The model under review builds one solid part; all positions refer to its coordinate system, in mm. A direction names the side the tool comes from. Coordinates: 2 decimals unless noted, no trailing zeros. Order: outer loops, then holes, each group sorted by start corner. A loop starts at its lowest first (then second) coordinate and runs counter-clockwise, first axis right, second up. Notation, with made-up numbers: M -19.75,-1.75 L 15.25,-1.75 A23 ccw 15.25,11.25 Z; hole C 87.25,44.25 d5. An arc over 180 degrees is marked long. Write each question's results on one line, items separated by ' | '.
from build123d import *

# Parameters (mm, degrees)
SKETCH1_W           = 170
SKETCH1_H           = 110
BOSS_EXTRUDE1_DEPTH = 30
FILLET2_R           = 10
FILLET3_R           = 10
FILLET4_R           = 10
SKETCH3_R           = 2.5
CUT_EXTRUDE1_DEPTH  = 5
CUT_EXTRUDE2_START  = -5
SKETCH5_R           = 2.5
CUT_EXTRUDE2_DEPTH  = 5
SKETCH6_W           = 3
SKETCH6_H           = 25
BOSS_EXTRUDE2_DEPTH = 25
SKETCH7_R           = 3.5
BOSS_EXTRUDE3_DEPTH = 4
SKETCH8_R           = 3.5
BOSS_EXTRUDE4_DEPTH = 4


with BuildPart() as part:
    # Sketch1 → Boss-Extrude1 (new body)
    with BuildSketch(Plane(origin=(0, 0, 0), x_dir=(1, 0, 0), z_dir=(0, 1, 0))):
        Rectangle(SKETCH1_W, SKETCH1_H)
    extrude(amount=BOSS_EXTRUDE1_DEPTH)

    # Fillet2
    fillet2_edges = [part.edges().sort_by_distance(p)[0] for p in [
        (-85, 30, 0),
        (0, 30, 55),
        (0, 0, 55),
        (85, 15, 55),
        (-85, 15, 55),
    ]]
    fillet(fillet2_edges, radius=FILLET2_R)

    # Fillet3
    # the kernel refuses this fillet: 10 mm, written as the material it takes off along each edge
    with BuildSketch(Plane(origin=(75, 20, 45), x_dir=(1, 0, 0), z_dir=(0, 1, 0))) as fillet3_piece_1_section:
        Polygon((0, 0), (FILLET3_R, 0), (FILLET3_R, -FILLET3_R), (0, -FILLET3_R), align=None)
    fillet3_piece_1 = extrude(amount=FILLET3_R, mode=Mode.PRIVATE)
    fillet3_piece_1 = fillet3_piece_1 - Plane(origin=(75, 20, 45), x_dir=(-0.7071067811865475, 0, -0.7071067811865475), z_dir=(0, 1, 0)) * Sphere(FILLET3_R, mode=Mode.PRIVATE)
    add(fillet3_piece_1, mode=Mode.SUBTRACT)
    with BuildSketch(Plane(origin=(75, 20, -45), x_dir=(0, 1, 0), z_dir=(0, 0, -1))) as fillet3_piece_2_section:
        Polygon((0, 0), (FILLET3_R, 0), (FILLET3_R, FILLET3_R), (0, FILLET3_R), align=None)
    fillet3_piece_2 = extrude(amount=FILLET3_R, mode=Mode.PRIVATE)
    fillet3_piece_2 = fillet3_piece_2 - Plane(origin=(75, 20, -45), x_dir=(-0.7071067811865475, -0.7071067811865475, 0), z_dir=(0, 0, -1)) * Sphere(FILLET3_R, mode=Mode.PRIVATE)
    add(fillet3_piece_2, mode=Mode.SUBTRACT)
    with BuildSketch(Plane(origin=(-85, -25, -55), x_dir=(1, 0, 0), z_dir=(0, 1, 0))) as fillet3_piece_3:
        with BuildLine():
            CenterArc((FILLET3_R, -FILLET3_R), FILLET3_R, 90, 90)
            Line((0, -FILLET3_R), (0, 0))
            Line((0, 0), (FILLET3_R, 0))
        make_face()
    extrude(amount=45, mode=Mode.SUBTRACT)
    with BuildSketch(Plane(origin=(85, 30, -45), x_dir=(-1, 0, 0), z_dir=(0, 0, 1))) as fillet3_piece_4:
        with BuildLine():
            CenterArc((FILLET3_R, FILLET3_R), FILLET3_R, 180, 90)
            Line((0, FILLET3_R), (0, 0))
            Line((0, 0), (FILLET3_R, 0))
        make_face()
    extrude(amount=90, mode=Mode.SUBTRACT)
    with BuildSketch(Plane(origin=(-75, 20, -55), x_dir=(-1, 0, 0), z_dir=(0, -1, 0))) as fillet3_piece_5:
        with BuildLine():
            CenterArc((10 - FILLET3_R, -FILLET3_R), FILLET3_R, 0, 90)
            Line((10, -FILLET3_R), (10, 0))
            Line((10, 0), (10 - FILLET3_R, 0))
        make_face()
    revolve(axis=Axis((-75, 20, -55), (0, 0, -1)), revolution_arc=90, mode=Mode.SUBTRACT)
    with BuildSketch(Plane(origin=(85, -25, -55), x_dir=(-1, 0, 0), z_dir=(0, 1, 0))) as fillet3_piece_6:
        with BuildLine():
            CenterArc((FILLET3_R, FILLET3_R), FILLET3_R, 180, 90)
            Line((0, FILLET3_R), (0, 0))
            Line((0, 0), (FILLET3_R, 0))
        make_face()
    extrude(amount=45, mode=Mode.SUBTRACT)
    with BuildSketch(Plane(origin=(-75, 30, -55), x_dir=(0, -1, 0), z_dir=(1, 0, 0))) as fillet3_piece_7:
        with BuildLine():
            CenterArc((FILLET3_R, -FILLET3_R), FILLET3_R, 90, 90)
            Line((0, -FILLET3_R), (0, 0))
            Line((0, 0), (FILLET3_R, 0))
        make_face()
    extrude(amount=150, mode=Mode.SUBTRACT)

    # Fillet4
    # the kernel refuses this fillet: 10 mm, written as the material it takes off along each edge
    with BuildSketch(Plane(origin=(75, 10, 45), x_dir=(1, 0, 0), z_dir=(0, -1, 0))) as fillet4_piece_1_section:
        Polygon((0, 0), (FILLET4_R, 0), (FILLET4_R, FILLET4_R), (0, FILLET4_R), align=None)
    fillet4_piece_1 = extrude(amount=FILLET4_R, mode=Mode.PRIVATE)
    fillet4_piece_1 = fillet4_piece_1 - Plane(origin=(75, 10, 45), x_dir=(-0.7071067811865475, 0, -0.7071067811865475), z_dir=(0, -1, 0)) * Sphere(FILLET4_R, mode=Mode.PRIVATE)
    add(fillet4_piece_1, mode=Mode.SUBTRACT)
    with BuildSketch(Plane(origin=(-75, 10, 45), x_dir=(-1, 0, 0), z_dir=(0, -1, 0))) as fillet4_piece_2_section:
        Polygon((0, 0), (FILLET4_R, 0), (FILLET4_R, -FILLET4_R), (0, -FILLET4_R), align=None)
    fillet4_piece_2 = extrude(amount=FILLET4_R, mode=Mode.PRIVATE)
    fillet4_piece_2 = fillet4_piece_2 - Plane(origin=(-75, 10, 45), x_dir=(0.7071067811865475, 0, -0.7071067811865475), z_dir=(0, -1, 0)) * Sphere(FILLET4_R, mode=Mode.PRIVATE)
    add(fillet4_piece_2, mode=Mode.SUBTRACT)
    with BuildSketch(Plane(origin=(85, 0, -45), x_dir=(-1, 0, 0), z_dir=(0, 0, 1)), Plane(origin=(-85, 0, 45), x_dir=(1, 0, 0), z_dir=(0, 0, -1))) as fillet4_piece_3:
        with BuildLine():
            CenterArc((FILLET4_R, -FILLET4_R), FILLET4_R, 90, 90)
            Line((0, -FILLET4_R), (0, 0))
            Line((0, 0), (FILLET4_R, 0))
        make_face()
    extrude(amount=90, mode=Mode.SUBTRACT)
    with BuildSketch(Plane(origin=(-75, 0, -55), x_dir=(0, 1, 0), z_dir=(1, 0, 0))) as fillet4_piece_4:
        with BuildLine():
            CenterArc((FILLET4_R, FILLET4_R), FILLET4_R, 180, 90)
            Line((0, FILLET4_R), (0, 0))
            Line((0, 0), (FILLET4_R, 0))
        make_face()
    extrude(amount=150, mode=Mode.SUBTRACT)
    with BuildSketch(Plane(origin=(75, 0, -45), x_dir=(0, 0, -1), z_dir=(-1, 0, 0))) as fillet4_piece_5:
        with BuildLine():
            CenterArc((10 - FILLET4_R, -FILLET4_R), FILLET4_R, 0, 90)
            Line((10, -FILLET4_R), (10, 0))
            Line((10, 0), (10 - FILLET4_R, 0))
        make_face()
    revolve(axis=Axis((75, 0, -45), (0, -1, 0)), revolution_arc=90, mode=Mode.SUBTRACT)
    with BuildSketch(Plane(origin=(-75, 0, -45), x_dir=(-1, 0, 0), z_dir=(0, 0, 1))) as fillet4_piece_6:
        with BuildLine():
            CenterArc((10 - FILLET4_R, -FILLET4_R), FILLET4_R, 0, 90)
            Line((10, -FILLET4_R), (10, 0))
            Line((10, 0), (10 - FILLET4_R, 0))
        make_face()
    revolve(axis=Axis((-75, 0, -45), (0, -1, 0)), revolution_arc=90, mode=Mode.SUBTRACT)

    # Sketch3 → Cut-Extrude1 (cut)
    with BuildSketch(Plane(origin=(0, 0, -55), x_dir=(-1, 0, 0), z_dir=(0, 0, -1))):
        with Locations((-66, 15)):
            Circle(SKETCH3_R)
        with Locations((66, 15)):
            Circle(SKETCH3_R)
    extrude(amount=-CUT_EXTRUDE1_DEPTH, mode=Mode.SUBTRACT)

    # Sketch5 → Cut-Extrude2 (cut)
    with BuildSketch(Plane.XY.offset(55).offset(CUT_EXTRUDE2_START)):
        with Locations(Location((-66, 15, 0), (0, 0, 180))):
            Circle(SKETCH5_R)
        with Locations(Location((66, 15, 0), (0, 0, 180))):
            Circle(SKETCH5_R)
    extrude(amount=CUT_EXTRUDE2_DEPTH, mode=Mode.SUBTRACT)

    # Sketch6 → Boss-Extrude2 (add)
    with BuildSketch(Plane(origin=(0, 30, 0), x_dir=(1, 0, 0), z_dir=(0, 1, 0))):
        with Locations((65, 30)):
            Rectangle(SKETCH6_W, SKETCH6_H)
        with Locations((65, -30)):
            Rectangle(SKETCH6_W, SKETCH6_H)
    extrude(amount=BOSS_EXTRUDE2_DEPTH)

    # Sketch7 → Boss-Extrude3 (add)
    with BuildSketch(Plane(origin=(66.5, 0, 0), x_dir=(0, 0, -1), z_dir=(1, 0, 0))):
        with Locations(Location((-30, 42.5, 0), (0, 0, 180))):
            Circle(SKETCH7_R)
    extrude(amount=BOSS_EXTRUDE3_DEPTH)

    # Sketch8 → Boss-Extrude4 (add)
    with BuildSketch(Plane(origin=(66.5, 0, 0), x_dir=(0, 0, -1), z_dir=(1, 0, 0))):
        with Locations(Location((30, 42.5, 0), (0, 0, 180))):
            Circle(SKETCH8_R)
    extrude(amount=BOSS_EXTRUDE4_DEPTH)


solid = part.part
1) Take a section at D-D on y = 6.5. State the section outline as (x, z) points (1 decimal), plus the area to 3 significant figures.
Solutions:
outline: M -84.4,-45 A9.4 ccw -75,-54.4 L 75,-54.4 A9.4 ccw 84.4,-45 L 84.4,45 A9.4 ccw 75,54.4 L -75,54.4 A9.4 ccw -84.4,45 Z | area: 18,300 mm2
2) For faces 1 (the flat face through (66, 15, 50)), 2 (the flat face through (70.5, 42, -30)), 3 (the cylindrical face through (68, 39, -30)), list the 3-axis set-ups (+Z, -Z, +X, -X, +Y, -Y) from which the entire face can be reached by the end or side of a thin tool; tool diameter is ignored.
Solutions:
face 1: +Z | face 2: +Z, -Z, +X, +Y | face 3: +X
3) To check wall thickness, follow line 1 along X through (y, z) = (15, 51.7); line 2 along Y through (x, z) = (20.5, -11); line 3 along X through (y, z) = (15, 52). State the ranges of each line that lie inside material, in increasing order.
Solutions:
line 1: -82.42 to -68.5, -63.5 to 63.5, 68.5 to 82.42 | line 2: 0 to 30 | line 3: -82.14 to -68.5, -63.5 to 63.5, 68.5 to 82.14
4) Take a section at C-C on x = 24. State the section outline as (y, z) points.
Solutions:
outline: M 0,-45 A10 ccw 10,-55 L 20,-55 A10 ccw 30,-45 L 30,45 A10 ccw 20,55 L 10,55 A10 ccw 0,45 Z
5) Take a section at B-B on z = 30. State the section outline as (x, y) points, plus the area to 3 significant figures.
Solutions:
outline: M -85,10 A10 ccw -75,0 L 75,0 A10 ccw 85,10 L 85,20 A10 ccw 75,30 L 66.5,30 L 66.5,39 L 70.5,39 L 70.5,46 L 66.5,46 L 66.5,55 L 63.5,55 L 63.5,30 L -75,30 A10 ccw -85,20 Z | area: 5,120 mm2
6) The part is to be moulded in two halves that separate along Y. For faces 4 (the cylindrical face through (-82.15, 26.99, -0.63)), 5 (the flat face through (66, 15, -50)), 6 (the flat face through (-1, 15, -55)), say which applies: pulls with the +Y half, pulls with the -Y half, needs draft (parallel to the pull), parting line crosses it, or undercut.
Solutions:
face 4: pulls with the +Y half | face 5: undercut | face 6: needs draft
7) For pin 1 (0.9 mm diameter, centred on x = 65, y = 42, fed in from -Z); pin 2 (3.5 mm diameter, centred on y = 42, z = -30.5, fed in from +X); pin 3 (7.5 mm diameter, centred on y = 45.5, z = -31.5, fed in from -X), all flat-tipped, find the tip position at first contact; note any pin that passes through.
Solutions:
pin 1: z = -42.5 | pin 2: x = 70.5 | pin 3: x = 63.5
8) Take a section at A-A on y = 37. State the section outline as (x, z) points, plus the area to 3 significant figures.
Solutions:
outline: M 63.5,-42.5 L 66.5,-42.5 L 66.5,-17.5 L 63.5,-17.5 Z; M 63.5,17.5 L 66.5,17.5 L 66.5,42.5 L 63.5,42.5 Z | area: 150 mm2
